Geometry check sheet. Reference: the model listing, model coordinates, mm. Coordinates: 2 decimals unless noted, no trailing zeros. Write each loop counter-clockwise with the first axis right and the second up, starting at its lowest first coordinate (ties: lowest second). Pieces come first, ordered by that corner, then holes. Notation, with made-up numbers: M 60.25,12 L 66.25,12 A27 ccw 66.25,31 Z; hole C -17,-37 d2. An arc over 180 degrees is marked long. Write each question's results on one line, items separated by ' | '.
```python
from build123d import *

# Parameters (mm, degrees)
SKETCH1_R           = 2.07
BOSS_EXTRUDE1_DEPTH = 0.875
FILLET1_R           = 2


with BuildPart() as part:
    # Sketch1 → Boss-Extrude1 (new, symmetric)
    with BuildSketch(Plane(origin=(0, 0, 0), x_dir=(1, 0, 0), z_dir=(0, 1, 0))):
        with BuildLine():
            ThreePointArc((-38.1, 11.43), (-49.53, 0), (-38.1, -11.43))
            Line((-38.1, -11.43), (38.1, -11.43))
            ThreePointArc((38.1, -11.43), (49.53, 0), (38.1, 11.43))
            Line((38.1, 11.43), (11.43, 11.43))
            Line((11.43, 11.43), (11.43, 38.1))
            ThreePointArc((11.43, 38.1), (0, 49.53), (-11.43, 38.1))
            Line((-11.43, 38.1), (-11.43, 11.43))
            Line((-11.43, 11.43), (-38.1, 11.43))
        make_face()
        with Locations(Location((-25.4, 0, 0), (0, 0, 270))):
            Circle(SKETCH1_R, mode=Mode.SUBTRACT)
        with Locations(Location((0, 25.4, 0), (0, 0, 270))):
            Circle(SKETCH1_R, mode=Mode.SUBTRACT)
        with Locations(Location((0, 12.7, 0), (0, 0, 270))):
            Circle(SKETCH1_R, mode=Mode.SUBTRACT)
        with Locations(Location((25.4, 0, 0), (0, 0, 270))):
            Circle(SKETCH1_R, mode=Mode.SUBTRACT)
        with Locations(Location((-12.7, 0, 0), (0, 0, 270))):
            Circle(SKETCH1_R, mode=Mode.SUBTRACT)
        with Locations(Location((0, 0, 0), (0, 0, 270))):
            Circle(SKETCH1_R, mode=Mode.SUBTRACT)
        with Locations(Location((12.7, 0, 0), (0, 0, 270))):
            Circle(SKETCH1_R, mode=Mode.SUBTRACT)
        with Locations(Location((-38.1, 0, 0), (0, 0, 270))):
            Circle(SKETCH1_R, mode=Mode.SUBTRACT)
        with Locations(Location((38.1, 0, 0), (0, 0, 270))):
            Circle(SKETCH1_R, mode=Mode.SUBTRACT)
        with Locations(Location((0, 38.1, 0), (0, 0, 270))):
            Circle(SKETCH1_R, mode=Mode.SUBTRACT)
    extrude(amount=BOSS_EXTRUDE1_DEPTH, both=True)

    # Fillet1
    fillet1_edges = [part.edges().sort_by_distance(p)[0] for p in [
        (11.43, 0, -11.43),
        (-11.43, 0, -11.43),
    ]]
    fillet(fillet1_edges, radius=FILLET1_R)


solid = part.part
```
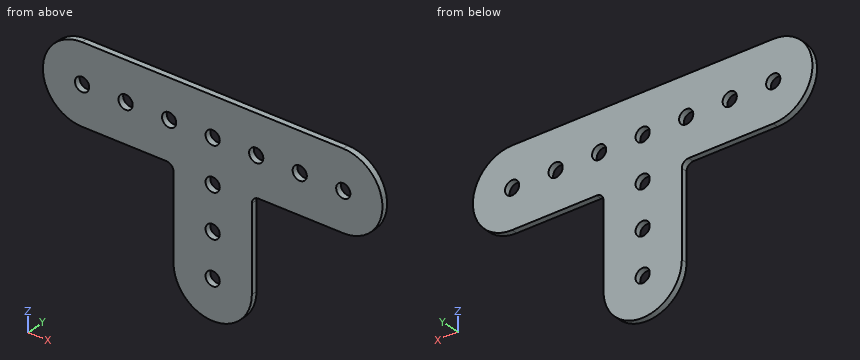
Q1. Sectioned sample at D-D on y = 0.45. Give the number of separate pieces and of enclosed holes in the cut face, and give its area (3 significant figures).
Geometry check:
separate pieces: 1 | enclosed holes: 10 | area: 2,830 mm2
Q2. Depth check by flat-ended pin: P1, Ø3.5, axis at x = 12.7, z = 0, coming from the +Y side; P2, Ø0.5, axis at y = -0.5, z = -24, coming from the -X side; P3, Ø0.9, axis at x = -31.5, y = 0, coming from the -Z side; P4, Ø0.9, axis at y = 0, z = -26.5, coming from the +X side. Enter the tip coordinate at first touch or a pass-through.
Geometry check:
P1: passes through | P2: stops at x = -11.43 | P3: stops at z = -11.43 | P4: stops at x = 11.43
Q3. Sectioned sample at C-C on z = -25.4. Record the cut outline in (x, y) (3 decimals), and give its area (3 significant figures).
Geometry check:
outline: M -11.43,-0.875 L -2.07,-0.875 L -2.07,0.875 L -11.43,0.875 Z; M 2.07,-0.875 L 11.43,-0.875 L 11.43,0.875 L 2.07,0.875 Z | area: 32.8 mm2
Q4. Scan lines: probe 1 along Z at (x, y) = (33, 0.2); probe 2 along Z at (x, y) = (14.5, 0.75). Record each from-to range of solid material in increasing order.
Geometry check:
probe 1: z = -11.43 to 11.43 | probe 2: z = -11.43 to -1.02, 1.02 to 11.43
Q5. Sectioned sample at A-A on x = 0. Record the cut outline in (y, z) (3 decimals), and give its area (3 significant figures).
Geometry check:
outline: M -0.875,-49.53 L 0.875,-49.53 L 0.875,-40.17 L -0.875,-40.17 Z; M -0.875,-36.03 L 0.875,-36.03 L 0.875,-27.47 L -0.875,-27.47 Z; M -0.875,-23.33 L 0.875,-23.33 L 0.875,-14.77 L -0.875,-14.77 Z; M -0.875,-10.63 L 0.875,-10.63 L 0.875,-2.07 L -0.875,-2.07 Z; M -0.875,2.07 L 0.875,2.07 L 0.875,11.43 L -0.875,11.43 Z | area: 77.7 mm2
Q6. Sectioned sample at B-B on x = -25.4. Record the cut outline in (y, z) (3 decimals).
Geometry check:
outline: M -0.875,-11.43 L 0.875,-11.43 L 0.875,-2.07 L -0.875,-2.07 Z; M -0.875,2.07 L 0.875,2.07 L 0.875,11.43 L -0.875,11.43 Z
